```python
from build123d import *

# Parameters (mm, degrees)
SKETCH1_R           = 12.7
BOSS_EXTRUDE1_DEPTH = 304.8
SKETCH2_R           = 3.96875
CUT_EXTRUDE1_DEPTH  = 76.2
SKETCH3_R           = 2.1971
CUT_EXTRUDE2_DEPTH  = 76.2


with BuildPart() as part:
    # Sketch1 → Boss-Extrude1 (new body)
    with BuildSketch(Plane(origin=(0, 0, 0), x_dir=(1, 0, 0), z_dir=(0, 1, 0))):
        with Locations(Location((0, 0, 0), (0, 0, 90))):
            Circle(SKETCH1_R)
    extrude(amount=BOSS_EXTRUDE1_DEPTH)

    # Sketch2 → Cut-Extrude1 (cut)
    with BuildSketch(Plane.XZ):
        with Locations(Location((0, 0, 0), (0, 0, 270))):
            Circle(SKETCH2_R)
    extrude(amount=-CUT_EXTRUDE1_DEPTH, mode=Mode.SUBTRACT)

    # Sketch3 → Cut-Extrude2 (cut)
    with BuildSketch(Plane(origin=(0, 304.8, 0), x_dir=(1, 0, 0), z_dir=(0, 1, 0))):
        with Locations(Location((0, 8.89, 0), (0, 0, 270))):
            Circle(SKETCH3_R)
        with Locations(Location((8.89, 0, 0), (0, 0, 270))):
            Circle(SKETCH3_R)
        with Locations(Location((0, -8.89, 0), (0, 0, 270))):
            Circle(SKETCH3_R)
        with Locations(Location((-8.89, 0, 0), (0, 0, 270))):
            Circle(SKETCH3_R)
    extrude(amount=-CUT_EXTRUDE2_DEPTH, mode=Mode.SUBTRACT)


solid = part.part
```
The listing builds one solid part. Answer for the finished solid, in the listing's coordinates (mm). Give positions to 0.01 mm unless a question says otherwise; leave off trailing zeros. Order: outer loops, then holes, each group sorted by start corner. A loop starts at its lowest first (then second) coordinate and runs counter-clockwise, first axis right, second up.
Item 1: The part is cut by section A-A, the plane y = 233. Give the vertices of the cut face in (x, z).
From the geometry:
outline: circle Ø25.4 at (0, 0); hole circle Ø4.39 at (-8.89, 0); hole circle Ø4.39 at (0, -8.89); hole circle Ø4.39 at (0, 8.89); hole circle Ø4.39 at (8.89, 0)
Item 2: For a pull along Z with two mould halves and no side action, classify faces 1 (the face through (0, 76.2, 0)), 2 (the face through (-3.874, 37.567, 0.86)), 3 (the face through (0, 304.8, 0)), 4 (the face through (7.7, 150.3, 10.1)) as pulls with the +Z half, pulls with the -Z half, needs draft (parallel to the pull), parting line crosses it, or undercut.
From the geometry:
face 1: undercut
face 2: undercut
face 3: needs draft
face 4: parting line crosses it
Item 3: The part is cut by section B-B, the plane y = 24. Give the vertices of the cut face in (x, z), and give its area (3 significant figures).
From the geometry:
outline: circle Ø25.4 at (0, 0); hole circle Ø7.94 at (0, 0)
area: 457 mm2
Item 4: Find the intervals of material crossed by probe 1 along X at (y, z) = (271.5, 0); probe 2 along X at (y, z) = (235, 1); probe 3 along Z at (x, y) = (9.5, 252.5), in increasing order.
From the geometry:
probe 1: x = -12.7 to -11.09, -6.69 to 6.69, 11.09 to 12.7
probe 2: x = -12.66 to -10.85, -6.93 to 6.93, 10.85 to 12.66
probe 3: z = -8.43 to -2.11, 2.11 to 8.43
Item 5: Given pin 1 Ø12 at (y, z) = (257.5, -9.5) entering from +X; pin 2 Ø3.5 at (x, z) = (-8.89, 0) entering from +Y; pin 3 Ø2 at (x, y) = (-7.5, 147.5) entering from +Z, each flat-ended and moving along its own axis, determine where each tip first touches the part or whether it passes through.
From the geometry:
pin 1: stops at x = 12.21
pin 2: stops at y = 228.6
pin 3: stops at z = 10.91
Item 6: The part is cut by section C-C, the plane y = 165.5. Give the vertices of the cut face in (x, z), and give its area (3 significant figures).
From the geometry:
outline: circle Ø25.4 at (0, 0)
area: 507 mm2
